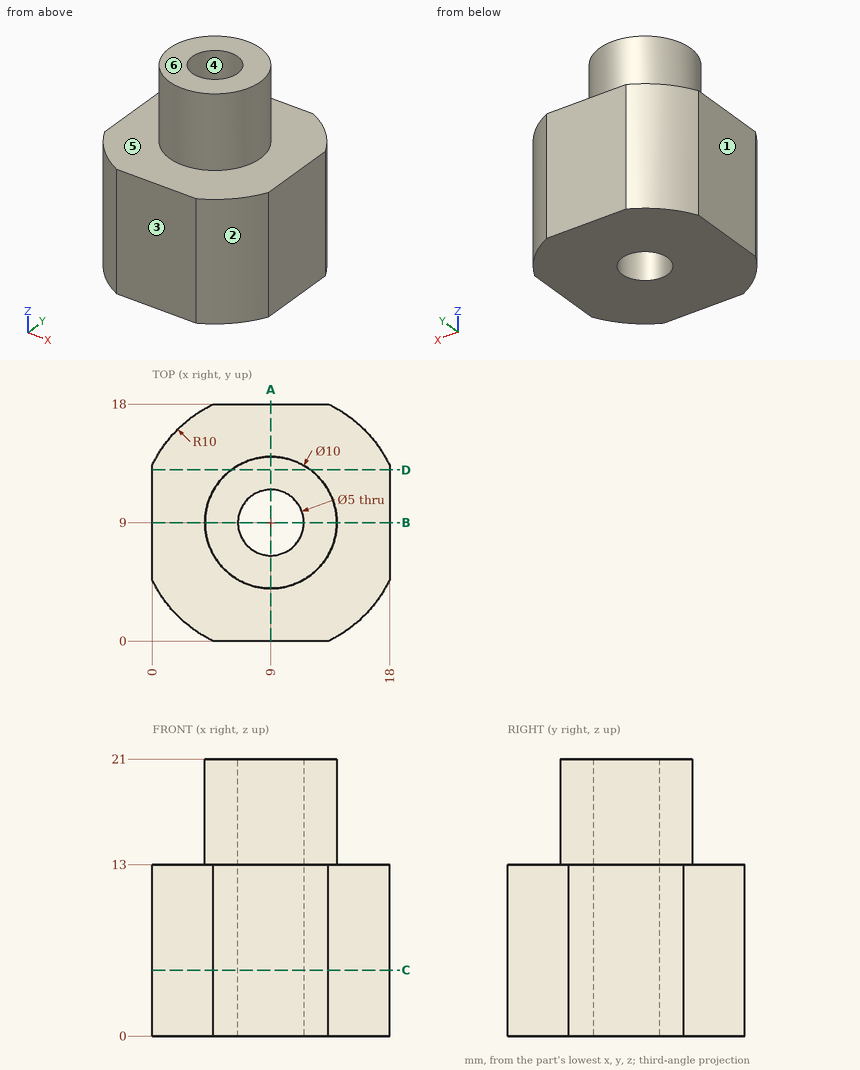
Here's the drawing with two shaded views (mm, measured from the low corner). I have some questions. A direction names the side the tool comes from. Coordinates: 2 decimals unless noted, no trailing zeros. Loops run counter-clockwise (first coordinate to the right, second up) from the corner with the lowest first, then second, coordinate; pieces in that order, holes last. Notation, with made-up numbers: M 18.25,71 L 53.25,71 A15 ccw 53.25,77 Z; hole C -4,2 d4. An arc over 180 degrees is marked long. Return JSON: item names as keys, results as strings. Group by question number.
Item 1: Thinking about a two-plate mould opening in X: for the marked faces 1, 2, 3 and 4, which applies, released by +X, released by -X, zero draft, split by the parting line, or undercut?
Item 2: On a 3-axis mill with a long thin cutter (end or side, diameter ignored), from which of +Z, -Z, +X, -X, +Y, -Y can I reach the whole of each face in a straight line? I mean the marked faces 5 and 6. Say none if no direction works.
Item 3: Imagine slicing it at D-D (y = 13). Please give me the cut outline in (x, z).
Item 4: I'm going to push flat-ended pins straight in: pin 1 Ø2 at (y, z) = (5, 17) entering from -X; pin 2 Ø5 at (x, z) = (15, 18) entering from -Y; pin 3 Ø5 at (y, z) = (11.5, 16.5) entering from -X. Where does each tip first touch, or does it pass through?
Item 5: Imagine slicing it at A-A (x = 9). Please give me the cut outline in (y, z).
Item 6: If I drill on L1, parallel to Y at x = 9, z = 10.5; L2, parallel to X at y = 9, z = 16.75, over which ranges is the centre line in solid material (lowest first)? Write a range as from..to.
Item 7: Imagine slicing it at C-C (z = 5). Please give me the cut outline in (x, y), and give its area (3 significant figures).
Verdict:
{
 "1": {"face 1": "released by -X", "face 2": "released by +X", "face 3": "zero draft", "face 4": "undercut"},
 "2": {"face 5": "+Z", "face 6": "+Z, +X, -X, +Y, -Y"},
 "3": {"outline": "M 0,0 L 18,0 L 18,13 L 12,13 L 12,21 L 6,21 L 6,13 L 0,13 Z"},
 "4": {"pin 1": "stops at x = 5", "pin 2": "stops at y = 5.43", "pin 3": "stops at x = 4"},
 "5": {"outline": "M 0,0 L 6.5,0 L 6.5,21 L 4,21 L 4,13 L 0,13 Z; M 11.5,0 L 18,0 L 18,13 L 14,13 L 14,21 L 11.5,21 Z"},
 "6": {"L1": "y = 0..6.5, 11.5..18", "L2": "x = 4..6.5, 11.5..14"},
 "7": {"outline": "M 0,4.64 A10 ccw 4.64,0 L 13.36,0 A10 ccw 18,4.64 L 18,13.36 A10 ccw 13.36,18 L 4.64,18 A10 ccw 0,13.36 Z; hole C 9,9 d5", "area": "271 mm^2"}
}
